```python
from build123d import *

# Parameters (mm, degrees)
PAD007_DEPTH = 50
SKETCH016_R  = 2.5
PAD008_DEPTH = 3.5
SKETCH017_R  = 2.5
PAD009_DEPTH = 3.5


with BuildPart() as part:
    # Sketch015 → Pad007 (new body)
    with BuildSketch(Plane.XY):
        with BuildLine():
            ThreePointArc((14.095389, 54.869698), (1.399981, 63.846416), (-14.095389, 65.130302))
            ThreePointArc((-14.095389, 65.130302), (-0.849311, 57.666538), (14.095389, 54.869698))
        make_face()
    extrude(amount=PAD007_DEPTH)

    # Sketch016 (on Face4 of Pad007) → Pad008 (join)
    with BuildSketch(Plane.XY.offset(50)):
        with Locations((0, 60)):
            Circle(SKETCH016_R)
    extrude(amount=PAD008_DEPTH)

    # Sketch017 (on Face3 of Pad008) → Pad009 (join)
    with BuildSketch(Plane(origin=(0, 0, 0), x_dir=(1, 0, 0), z_dir=(0, 0, -1))):
        with Locations((0, -60)):
            Circle(SKETCH017_R)
    extrude(amount=PAD009_DEPTH)


solid = part.part
```
Work out the finished part from the listing and answer in its coordinate system (mm). A direction names the side the tool comes from. Coordinates: 2 decimals unless noted, no trailing zeros. Write each loop counter-clockwise with the first axis right and the second up, starting at its lowest first coordinate (ties: lowest second). Pieces come first, ordered by that corner, then holes.
Q1. Which of the six approach directions +Z, -Z, +X, -X, +Y, -Y give full straight-line access (tool end or side, diameter ignored) to faces 1 (the face through (0, 60, 53.5)), 2 (the face through (1.34, 57.89, -1.73))?
Q2. Determine the mould class of faces 3 (the face through (-0.54, 57.56, 51.73)), 4 (the face through (-1.05, 57.74, 24.65)), 5 (the face through (0, 63, 50)) for opening direction X: released by +X, released by -X, zero draft, split by the parting line, or undercut.
Q3. A cutting plane is placed at D-D, the plane y = 64.5. Give the vertices of the cut face in (x, z).
Q4. A cutting plane is placed at A-A, the plane x = 1. Give the vertices of the cut face in (y, z), then the cut area to 3 significant figures.
Q5. A cutting plane is placed at C-C, the plane z = 9.5. Give the vertices of the cut face in (x, y), then the cut area to 3 significant figures.
Q6. Each of these flat-tipped pins is pushed along its axis until it touches: pin 1 Ø5 at (y, z) = (61.5, 43) entering from +X; pin 2 Ø1 at (x, z) = (9.5, 20.5) entering from -Y; pin 3 Ø5 at (x, y) = (-10.5, 59.5) entering from +Z; pin 4 Ø2 at (y, z) = (63.5, 2.5) entering from -X. Where does it stop, or does it pass through?
Q7. Find the intervals of material crossed by line 1 (Z direction, x = -3.5, y = 63.5); line 2 (X direction, y = 63, z = 36.5); line 3 (X direction, y = 58.5, z = 45.5), in increasing order.
Q8. A cutting plane is placed at B-B, the plane y = 60. Give the vertices of the cut face in (x, z), then the cut area to 3 significant figures.
Findings below:
1. face 1: +Z, +X, -X, +Y, -Y
1. face 2: -Z
2. face 3: split by the parting line
2. face 4: released by -X
2. face 5: zero draft
3. outline: (-13.29, 0) - (-0.62, 0) - (-0.62, 50) - (-13.29, 50) - close
4. outline: (57.04, 0) - (57.71, 0) - (57.71, -3.5) - (62.29, -3.5) - (62.29, 0) - (63.99, 0) - (63.99, 50) - (62.29, 50) - (62.29, 53.5) - (57.71, 53.5) - (57.71, 50) - (57.04, 50) - close
4. area: 380 mm2
5. outline: (-14.1, 65.13) arc R46.55 ccw to (14.1, 54.87) arc R29.53 ccw to start
5. area: 133 mm2
6. pin 1: stops at x = 9.94
6. pin 2: stops at y = 55.14
6. pin 3: passes through
6. pin 4: stops at x = -13.29
7. line 1: z = 0 to 50
7. line 2: x = -11.23 to 3.48
7. line 3: x = -2.98 to 10.54
8. outline: (-6.19, 0) - (-2.5, 0) - (-2.5, -3.5) - (2.5, -3.5) - (2.5, 0) - (8.64, 0) - (8.64, 50) - (2.5, 50) - (2.5, 53.5) - (-2.5, 53.5) - (-2.5, 50) - (-6.19, 50) - close
8. area: 777 mm2
